from build123d import *

# Parameters (mm, degrees)
SKETCH1_R                = 101.6
BOSS_EXTRUDE1_DEPTH      = 38.1
BOSS_EXTRUDE1_DEPTH_BACK = 38.1
SKETCH2_R                = 12.7
CUT_EXTRUDE1_DEPTH       = 77.2
FILLET1_R                = 12.7
FILLET2_R                = 12.7
CUT_EXTRUDE2_DEPTH       = 77.2


with BuildPart() as part:
    # Sketch1 → Boss-Extrude1 (new body, two sides)
    with BuildSketch(Plane.XY) as boss_extrude1_sk:
        Circle(SKETCH1_R)
    extrude(amount=BOSS_EXTRUDE1_DEPTH)
    extrude(boss_extrude1_sk.sketch, amount=-BOSS_EXTRUDE1_DEPTH_BACK)

    # Sketch2 → Cut-Extrude1 (cut, through all)
    with BuildSketch(Plane.XY.offset(38.1)):
        Circle(SKETCH2_R)
    extrude(amount=-CUT_EXTRUDE1_DEPTH, mode=Mode.SUBTRACT)

    # Fillet1
    fillet1_edges = [part.edges().sort_by_distance(p)[0] for p in [
        (-101.6, 0, 38.1),
    ]]
    fillet(fillet1_edges, radius=FILLET1_R)

    # Fillet2
    fillet2_edges = [part.edges().sort_by_distance(p)[0] for p in [
        (-101.6, 0, -38.1),
    ]]
    fillet(fillet2_edges, radius=FILLET2_R)

    # Sketch3 → Cut-Extrude2 (cut, through all)
    with BuildSketch(Plane.XY.offset(38.1)):
        with BuildLine():
            Line((5.110599479, 24.880550094), (16.107968661, 74.486476782))
            ThreePointArc((16.107968661, 74.486476782), (-0.197840063, 76.208022787), (-16.494490613, 74.401839071))
            Line((-16.494490613, 74.401839071), (-5.497566194, 24.797918581))
            ThreePointArc((-5.497566194, 24.797918581), (-0.197845398, 25.399229461), (5.110599479, 24.880550094))
        make_face()
    cut_extrude2 = extrude(amount=-CUT_EXTRUDE2_DEPTH, mode=Mode.SUBTRACT)

    # Mirror1: Cut-Extrude2 across plane
    add(cut_extrude2.mirror(Plane.ZX), mode=Mode.SUBTRACT)


solid = part.part
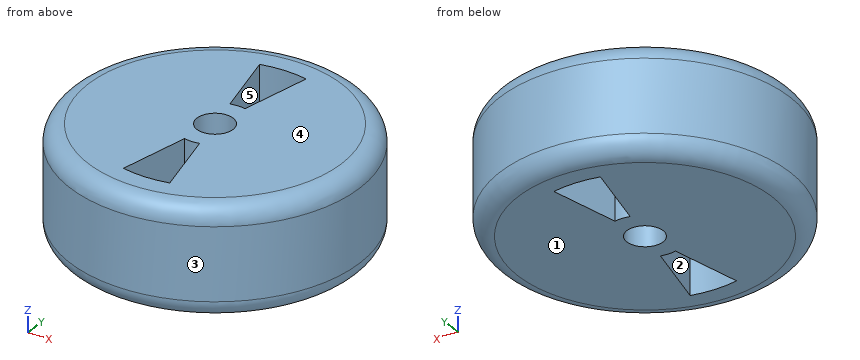
Build history of the part. All positions in model axes, mm. Face numbers are marked on the shaded views. A direction names the side the tool comes from. Coordinates: 2 decimals unless noted, no trailing zeros. Write each loop counter-clockwise with the first axis right and the second up, starting at its lowest first coordinate (ties: lowest second). Pieces come first, ordered by that corner, then holes.
(1) 3-axis set-ups, long thin cutter, end or side, ignore diameter. For the marked faces 1 and 2: which of +Z, -Z, +X, -X, +Y, -Y reach the whole face in a straight line?
(2) Mould opens along X. For the marked faces 3, 4 and 5 say: pulls with the +X half, pulls with the -X half, needs draft (parallel to the pull), parting line crosses it, or undercut.
(3) Cut at D-D on z = -33. List the corners of the cut face in (x, y), and give its area (3 significant figures).
(4) Drill centre lines: line 1 (Y direction, x = 0, z = 13.5); line 2 (X direction, y = 66, z = 5); line 3 (X direction, y = -34, z = -29.5). Where is each one in solid material? Low to high.
(5) Cut at B-B on y = 0. List the corners of the cut face in (x, z).
(6) Pin check, flat tips, straight feed: pin 1 Ø6 at (y, z) = (77, -7.5) entering from +X; pin 2 Ø8 at (y, z) = (61.5, -21.5) entering from +X; pin 3 Ø1.5 at (y, z) = (-73, 6) entering from +X. Stop position of each tip, or through.
(7) Cut at C-C on z = 15. List the corners of the cut face in (x, y).
(8) Cut at A-A on x = 0. List the corners of the cut face in (y, z).
Working result:
1. face 1: -Z, +X, -X, +Y, -Y
1. face 2: +Z, -Z
2. face 3: parting line crosses it
2. face 4: needs draft
2. face 5: undercut
3. outline: circle Ø198.15 at (0, 0); hole (-16.49, -74.4) arc R76.21 ccw to (16.11, -74.49) - (5.11, -24.88) arc R25.4 cw to (-5.5, -24.8) - close; hole (-16.49, 74.4) - (-5.5, 24.8) arc R25.4 cw to (5.11, 24.88) - (16.11, 74.49) arc R76.21 ccw to start; hole circle Ø25.4 at (0, 0)
3. area: 28,100 mm2
4. line 1: y = -101.6 to -76.21, -25.4 to -12.7, 12.7 to 25.4, 76.21 to 101.6
4. line 2: x = -77.24 to -14.63, 14.23 to 77.24
4. line 3: x = -95.02 to -7.54, 7.13 to 95.02
5. outline: (-101.6, -25.4) arc R12.7 ccw to (-88.9, -38.1) - (-12.7, -38.1) - (-12.7, 38.1) - (-88.9, 38.1) arc R12.7 ccw to (-101.6, 25.4) - close; (12.7, -38.1) - (88.9, -38.1) arc R12.7 ccw to (101.6, -25.4) - (101.6, 25.4) arc R12.7 ccw to (88.9, 38.1) - (12.7, 38.1) - close
6. pin 1: stops at x = 69.62
6. pin 2: stops at x = 83.76
6. pin 3: stops at x = 71.43
7. outline: circle Ø203.2 at (0, 0); hole (-16.49, -74.4) arc R76.21 ccw to (16.11, -74.49) - (5.11, -24.88) arc R25.4 cw to (-5.5, -24.8) - close; hole (-16.49, 74.4) - (-5.5, 24.8) arc R25.4 cw to (5.11, 24.88) - (16.11, 74.49) arc R76.21 ccw to start; hole circle Ø25.4 at (0, 0)
8. outline: (-101.6, -25.4) arc R12.7 ccw to (-88.9, -38.1) - (-76.21, -38.1) - (-76.21, 38.1) - (-88.9, 38.1) arc R12.7 ccw to (-101.6, 25.4) - close; (-25.4, -38.1) - (-12.7, -38.1) - (-12.7, 38.1) - (-25.4, 38.1) - close; (12.7, -38.1) - (25.4, -38.1) - (25.4, 38.1) - (12.7, 38.1) - close; (76.21, -38.1) - (88.9, -38.1) arc R12.7 ccw to (101.6, -25.4) - (101.6, 25.4) arc R12.7 ccw to (88.9, 38.1) - (76.21, 38.1) - close
